Read the model definition and answer for the solid it produces. Units are mm, in the model's axes. Face numbers are marked on the shaded views. A direction names the side the tool comes from. Coordinates: 2 decimals unless noted, no trailing zeros. Loops run counter-clockwise (first coordinate to the right, second up) from the corner with the lowest first, then second, coordinate; pieces in that order, holes last.
Q1. Which of the six approach directions +Z, -Z, +X, -X, +Y, -Y give full straight-line access (tool end or side, diameter ignored) to the marked faces 5 and 6?
Q2. Flat-ended cylindrical pins translate along their axes: P1, Ø2.5, axis at x = 12.5, z = 12.5, coming from the +Y side; P2, Ø3, axis at y = 10, z = 0, coming from the +X side. Find the tip coordinate at first contact, or state that the pin passes through.
Q3. The mould has two halves that part along Z. Classify the marked faces 1, 2, 3 and 4: pulls with the +Z half, pulls with the -Z half, needs draft (parallel to the pull), parting line crosses it, or undercut.
Q4. Section A-A (y = 13.5) is taken. Give the vertices of the cut face in (x, z).
Q5. Straight lines are drawn through the part: line 1 (Z direction, x = 12.5, y = 7); line 2 (Z direction, x = 0, y = 11). For each, find the intervals that lie inside material, in ascending order.
Q6. Section B-B (y = 2) is taken. Give the vertices of the cut face in (x, z).
from build123d import *

# Parameters (mm, degrees)
SKETCH1_W              = 35
SKETCH1_H              = 35
BOSS_EXTRUDE1_DEPTH    = 20
SKETCH2_R              = 10
BOSS_EXTRUDE2_DEPTH    = 1
M14_TAPPED_HOLE1_D     = 12
M14_TAPPED_HOLE1_DEPTH = 14
M14_TAPPED_HOLE1_TIP   = 3.605163714
M4_TAPPED_HOLE1_D      = 3.3
M4_TAPPED_HOLE1_DEPTH  = 10.1
M4_TAPPED_HOLE1_TIP    = 0.991420021
M4_TAPPED_HOLE2_D      = 3.3
M4_TAPPED_HOLE2_DEPTH  = 9
M4_TAPPED_HOLE2_TIP    = 0.991420021
CHAMFER1_SIZE          = 3
CHAMFER2_SIZE          = 0.5


with BuildPart() as part:
    # Sketch1 → Boss-Extrude1 (new body)
    with BuildSketch(Plane(origin=(0, 0, 0), x_dir=(1, 0, 0), z_dir=(0, 1, 0))):
        Rectangle(SKETCH1_W, SKETCH1_H)
    extrude(amount=BOSS_EXTRUDE1_DEPTH)

    # Sketch2 → Boss-Extrude2 (add)
    with BuildSketch(Plane(origin=(0, 20, 0), x_dir=(1, 0, 0), z_dir=(0, 1, 0))):
        with Locations(Location((0, 0, 0), (0, 0, 270))):
            Circle(SKETCH2_R)
    extrude(amount=BOSS_EXTRUDE2_DEPTH)

    # M14 Tapped Hole1
    with Locations(Plane(origin=(0, 21, 0), x_dir=(1, 0, 0), z_dir=(0, 1, 0))):
        with Locations((0, 0)):
            Hole(M14_TAPPED_HOLE1_D / 2, depth=M14_TAPPED_HOLE1_DEPTH)
            with Locations((0, 0, -(M14_TAPPED_HOLE1_DEPTH + M14_TAPPED_HOLE1_TIP / 2))):  # 118° drill point
                Cone(0, M14_TAPPED_HOLE1_D / 2, M14_TAPPED_HOLE1_TIP, mode=Mode.SUBTRACT)

    # M4 Tapped Hole1
    with Locations(Plane(origin=(0, 0, 0), x_dir=(-1, 0, 0), z_dir=(0, -1, 0))):
        with Locations((-12.5, 12.5), (-12.5, -12.5), (12.5, -12.5), (12.5, 12.5)):
            Hole(M4_TAPPED_HOLE1_D / 2, depth=M4_TAPPED_HOLE1_DEPTH)
            with Locations((0, 0, -(M4_TAPPED_HOLE1_DEPTH + M4_TAPPED_HOLE1_TIP / 2))):  # 118° drill point
                Cone(0, M4_TAPPED_HOLE1_D / 2, M4_TAPPED_HOLE1_TIP, mode=Mode.SUBTRACT)

    # M4 Tapped Hole2
    with Locations(Plane(origin=(17.5, 0, 0), x_dir=(0, 0, -1), z_dir=(1, 0, 0))):
        with Locations((0, 10)):
            Hole(M4_TAPPED_HOLE2_D / 2, depth=M4_TAPPED_HOLE2_DEPTH)
            with Locations((0, 0, -(M4_TAPPED_HOLE2_DEPTH + M4_TAPPED_HOLE2_TIP / 2))):  # 118° drill point
                Cone(0, M4_TAPPED_HOLE2_D / 2, M4_TAPPED_HOLE2_TIP, mode=Mode.SUBTRACT)

    # Chamfer1
    chamfer1_edges = [part.edges().sort_by_distance(p)[0] for p in [
        (-17.5, 10, -17.5),
        (17.5, 10, -17.5),
        (17.5, 10, 17.5),
        (-17.5, 10, 17.5),
    ]]
    chamfer(chamfer1_edges, length=CHAMFER1_SIZE)

    # Chamfer2
    chamfer2_edges = [part.edges().sort_by_distance(p)[0] for p in [
        (0, 21, -10),
    ]]
    chamfer(chamfer2_edges, length=CHAMFER2_SIZE)


solid = part.part
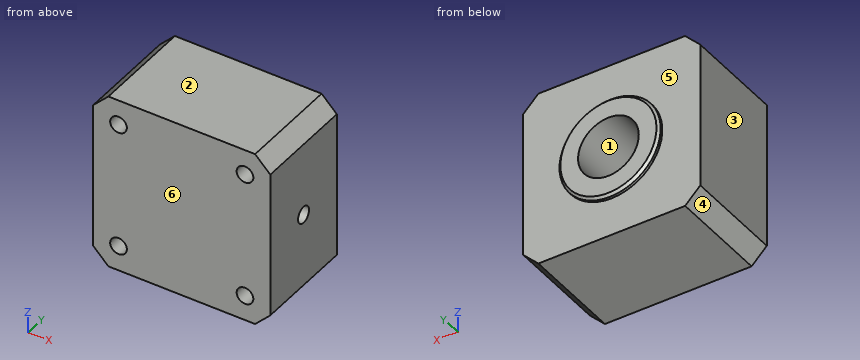
Numbers:
1. face 5: +Y
1. face 6: +Z, -Z, +X, -X, -Y
2. P1: stops at y = 20
2. P2: stops at x = 8.41
3. face 1: undercut
3. face 2: pulls with the +Z half
3. face 3: needs draft
3. face 4: pulls with the -Z half
4. outline: (-17.5, -14.5) - (-14.5, -17.5) - (14.5, -17.5) - (17.5, -14.5) - (17.5, 14.5) - (14.5, 17.5) - (-14.5, 17.5) - (-17.5, 14.5) - close; hole circle Ø12 at (0, 0)
5. line 1: z = -17.5 to -14.15, -10.85 to 10.85, 14.15 to 17.5
5. line 2: z = -17.5 to -6, 6 to 17.5
6. outline: (-17.5, -14.5) - (-14.5, -17.5) - (14.5, -17.5) - (17.5, -14.5) - (17.5, 14.5) - (14.5, 17.5) - (-14.5, 17.5) - (-17.5, 14.5) - close; hole circle Ø3.3 at (-12.5, -12.5); hole circle Ø3.3 at (-12.5, 12.5); hole circle Ø3.3 at (12.5, -12.5); hole circle Ø3.3 at (12.5, 12.5)
